from build123d import *

# Parameters (mm, degrees)
ESQUISSE1_R                                         = 18
BOSS_EXTRU_1_DEPTH                                  = 40
SKETCH1_R                                           = 20
BOSS_EXTRUDE1_DEPTH                                 = 2
CBORE_FOR_M3_HEX_SOCKET_HEAD_CAP_SCREW1_D           = 3.4
CBORE_FOR_M3_HEX_SOCKET_HEAD_CAP_SCREW1_CBORE_D     = 6.5
CBORE_FOR_M3_HEX_SOCKET_HEAD_CAP_SCREW1_CBORE_DEPTH = 3.4
ESQUISSE5_R                                         = 9.5
ENL_V_MAT_EXTRU_1_DEPTH                             = 35
ESQUISSE6_R                                         = 8
CUT_EXTRUDE2_DEPTH                                  = 41
CHAMFER1_SIZE                                       = 0.5


with BuildPart() as part:
    # Esquisse1 → Boss.-Extru.1 (new body)
    with BuildSketch(Plane.XY):
        Circle(ESQUISSE1_R)
    extrude(amount=BOSS_EXTRU_1_DEPTH)

    # Sketch1 → Boss-Extrude1 (add)
    with BuildSketch(Plane.XY.offset(40)):
        Circle(SKETCH1_R)
    extrude(amount=-BOSS_EXTRUDE1_DEPTH)

    # CBORE for M3 Hex Socket Head Cap Screw1 (through all)
    with Locations(Plane(origin=(0, 0, 0), x_dir=(-1, 0, 0), z_dir=(0, 0, -1))):
        with Locations((-8.838834765, -8.838834765), (-8.838834765, 8.838834765), (8.838834765, -8.838834765), (8.838834765, 8.838834765), (0, 0)):
            CounterBoreHole(CBORE_FOR_M3_HEX_SOCKET_HEAD_CAP_SCREW1_D / 2, CBORE_FOR_M3_HEX_SOCKET_HEAD_CAP_SCREW1_CBORE_D / 2, CBORE_FOR_M3_HEX_SOCKET_HEAD_CAP_SCREW1_CBORE_DEPTH)

    # Esquisse5 → Enlèv. mat.-Extru.1 (cut)
    with BuildSketch(Plane.XY.offset(40)):
        Circle(ESQUISSE5_R)
    extrude(amount=-ENL_V_MAT_EXTRU_1_DEPTH, mode=Mode.SUBTRACT)

    # Esquisse6 → Cut-Extrude2 (cut, through all)
    with BuildSketch(Plane(origin=(0, 0, 0), x_dir=(-1, 0, 0), z_dir=(0, 0, -1))):
        Circle(ESQUISSE6_R)
    extrude(amount=-CUT_EXTRUDE2_DEPTH, mode=Mode.SUBTRACT)

    # Chamfer1
    chamfer1_edges = [part.edges().sort_by_distance(p)[0] for p in [
        (-18, 0, 0),
    ]]
    chamfer(chamfer1_edges, length=CHAMFER1_SIZE)


solid = part.part
Design review of the part built by this model. Coordinates are the model's own, in mm. A direction names the side the tool comes from. Coordinates: 2 decimals unless noted, no trailing zeros. Loops run counter-clockwise (first coordinate to the right, second up) from the corner with the lowest first, then second, coordinate; pieces in that order, holes last. Notation, with made-up numbers: (-15.75, 30) - (2.25, 30) arc R10 ccw to (2.25, 46) - close; hole circle Ø10 at (47.5, -8.75). An arc over 180 degrees is marked (long way). Use CSV: the item, a comma, the result in double quotes. Start each with the question number.
1. For faces 1 (the cylindrical face through (8.47, 7.18, 21.96)), 2 (the flat face through (-4.3, -7, 5)), 3 (the flat face through (-18, 3, 38)), list the 3-axis set-ups (+Z, -Z, +X, -X, +Y, -Y) from which the entire face can be reached by the end or side of a thin tool; tool diameter is ignored.
2. Add section C-C on z = 31. Give the boundary of the cut face in (x, y), plus the area to 3 significant figures.
3. Mouldability with a two-part tool opening along Y and no side actions: class faces 4 (the cylindrical face through (-4.336, -19.524, 39.014)), 5 (the cylindrical face through (1.73, -7.81, 2.46)), 6 (the flat face through (4, -9, 40)) as released by +Y, released by -Y, zero draft, split by the parting line, or undercut.
4. Clearance check with flat-ended pins moving along their axes: pin 1 (12 mm diameter, centred on x = 1.5, z = 29.5, fed in from +Y); pin 2 (1.5 mm diameter, centred on y = 2.5, z = 32, fed in from -X); pin 3 (1.5 mm diameter, centred on x = -13, z = 9.5, fed in from +Y); pin 4 (3 mm diameter, centred on x = 8.84, y = 8.84, fed in from -Z) (1 decimal). State where each tip first meets the part, or that it passes through.
5. Add section A-A on y = 0. Give the boundary of the cut face in (x, z), plus the area to 3 significant figures.
6. To check wall thickness, follow probe 1 along Y at (x, z) = (-0.5, 19); probe 2 along Z at (x, y) = (17, -7); probe 3 along Z at (x, y) = (11.5, -9). State the ranges of each line that lie inside material, in increasing order.
Resolved:
1,face 1,"+Z, -Z"
1,face 2,"+Z"
1,face 3,"-Z"
2,outline,"circle Ø36 at (0, 0); hole circle Ø3.4 at (-8.84, -8.84); hole circle Ø3.4 at (-8.84, 8.84); hole circle Ø19 at (0, 0); hole circle Ø3.4 at (8.84, -8.84); hole circle Ø3.4 at (8.84, 8.84)"
2,area,"698 mm2"
3,face 4,"split by the parting line"
3,face 5,"undercut"
3,face 6,"zero draft"
4,pin 1,"y = 18"
4,pin 2,"x = -17.91"
4,pin 3,"y = 13.19"
4,pin 4,"through"
5,outline,"(-20, 38) - (-18, 38) - (-18, 0.5) - (-17.5, 0) - (-8, 0) - (-8, 5) - (-9.5, 5) - (-9.5, 40) - (-20, 40) - close; (8, 0) - (17.5, 0) - (18, 0.5) - (18, 38) - (20, 38) - (20, 40) - (9.5, 40) - (9.5, 5) - (8, 5) - close"
5,area,"703 mm2"
6,probe 1,"-17.99 to -9.49, 9.49 to 17.99"
6,probe 2,"38 to 40"
6,probe 3,"3.4 to 40"
